Source: CAD feature listing. Evaluate the final solid. Frame: model axes, mm. A direction names the side the tool comes from. Round coordinates to 2 decimals unless told otherwise and drop trailing zeros. Loops run counter-clockwise (first coordinate to the right, second up) from the corner with the lowest first, then second, coordinate; pieces in that order, holes last. Notation, with made-up numbers: M 11.25,84.5 L 60.25,84.5 A23 ccw 60.25,99.5 Z; hole C 86.5,19 d6. An arc over 180 degrees is marked long. Answer as CSV lines item,"result". Start each with the question number.
```python
from build123d import *

# Parameters (mm, degrees)
SKETCH2_W           = 51.27
SKETCH2_H           = 26.65
BOSS_EXTRUDE2_DEPTH = 5
SKETCH3_W           = 45.27
SKETCH3_H           = 20.65
CUT_EXTRUDE1_DEPTH  = 6
SKETCH4_W           = 3.75
SKETCH4_H           = 3.75
BOSS_EXTRUDE3_DEPTH = 5
SKETCH5_R           = 1.12
CUT_EXTRUDE2_DEPTH  = 6
SKETCH6_W           = 15
SKETCH6_H           = 57.7
BOSS_EXTRUDE4_DEPTH = 5
SKETCH7_W           = 25.4
SKETCH7_H           = 9.5
BOSS_EXTRUDE5_DEPTH = 5
SKETCH11_R          = 1.75
CUT_EXTRUDE5_DEPTH  = 6
SKETCH12_W          = 25.4
SKETCH12_H          = 0.2
CUT_EXTRUDE6_DEPTH  = 6


with BuildPart() as part:
    # Sketch2 → Boss-Extrude2 (new body)
    with BuildSketch(Plane(origin=(0, 0, 0), x_dir=(1, 0, 0), z_dir=(0, 1, 0))):
        with Locations((22.635, 10.325)):
            Rectangle(SKETCH2_W, SKETCH2_H)
    extrude(amount=BOSS_EXTRUDE2_DEPTH)

    # Sketch3 → Cut-Extrude1 (cut, through all)
    with BuildSketch(Plane(origin=(0, 5, 0), x_dir=(1, 0, 0), z_dir=(0, 1, 0))):
        with Locations((22.635, 10.325)):
            Rectangle(SKETCH3_W, SKETCH3_H)
    extrude(amount=-CUT_EXTRUDE1_DEPTH, mode=Mode.SUBTRACT)

    # Sketch4 → Boss-Extrude3 (add)
    with BuildSketch(Plane(origin=(0, 5, 0), x_dir=(1, 0, 0), z_dir=(0, 1, 0))):
        with Locations((1.875, 18.775)):
            Rectangle(SKETCH4_W, SKETCH4_H)
        with Locations((1.875, 1.875)):
            Rectangle(SKETCH4_W, SKETCH4_H)
        with Locations((43.395, 1.875)):
            Rectangle(SKETCH4_W, SKETCH4_H)
        with Locations((43.395, 18.775)):
            Rectangle(SKETCH4_W, SKETCH4_H)
    extrude(amount=-BOSS_EXTRUDE3_DEPTH)

    # Sketch5 → Cut-Extrude2 (cut, through all)
    with BuildSketch(Plane(origin=(0, 5, 0), x_dir=(1, 0, 0), z_dir=(0, 1, 0))):
        with Locations((1.385, 18.975)):
            Circle(SKETCH5_R)
        with Locations((43.885, 18.975)):
            Circle(SKETCH5_R)
        with Locations((43.885, 1.675)):
            Circle(SKETCH5_R)
        with Locations((1.385, 1.675)):
            Circle(SKETCH5_R)
    extrude(amount=-CUT_EXTRUDE2_DEPTH, mode=Mode.SUBTRACT)

    # Sketch6 → Boss-Extrude4 (add)
    with BuildSketch(Plane(origin=(0, 5, 0), x_dir=(1, 0, 0), z_dir=(0, 1, 0))):
        with Locations((22.635, -31.85)):
            Rectangle(SKETCH6_W, SKETCH6_H)
    extrude(amount=-BOSS_EXTRUDE4_DEPTH)

    # Sketch7 → Boss-Extrude5 (add)
    with BuildSketch(Plane(origin=(0, 5, 0), x_dir=(1, 0, 0), z_dir=(0, 1, 0))):
        with Locations((22.635, -65.45)):
            Rectangle(SKETCH7_W, SKETCH7_H)
    extrude(amount=-BOSS_EXTRUDE5_DEPTH)

    # Sketch11 → Cut-Extrude5 (cut, through all)
    with BuildSketch(Plane.XZ):
        with Locations((30.335, 65.51777032)):
            Circle(SKETCH11_R)
        with Locations((14.935, 65.51777032)):
            Circle(SKETCH11_R)
    extrude(amount=-CUT_EXTRUDE5_DEPTH, mode=Mode.SUBTRACT)

    # Sketch12 → Cut-Extrude6 (cut, through all)
    with BuildSketch(Plane(origin=(0, 5, 0), x_dir=(1, 0, 0), z_dir=(0, 1, 0))):
        with Locations((22.635, -70.1)):
            Rectangle(SKETCH12_W, SKETCH12_H)
    extrude(amount=-CUT_EXTRUDE6_DEPTH, mode=Mode.SUBTRACT)


solid = part.part
```
1) Section C-C, the plane x = 40.5. Return loops of the section in (y, z), and give its area (3 significant figures).
2) Ray query, line 1 along Z through (x, y) = (10, 2.4); line 2 along Z through (x, y) = (4.5, 4.2); line 3 along Z through (x, y) = (3, 0.95). Return the intervals inside material, ascending.
3) Section A-A, the plane x = 26.5. Return loops of the section in (y, z), and give its area (3 significant figures).
4) Mould query, pull axis X, two halves, no side actions, for faces 5 (the flat face through (3.75, 3, -2)), 6 (the cylindrical face through (1.239, 2.535, -20.085)), 7 (the flat face through (22, 0, 23)), 8 (the flat face through (30.135, 3, 32)). Classes: pulls with the +X half, pulls with the -X half, needs draft (parallel to the pull), parting line crosses it, or undercut.
5) Contact query for flat-ended pins moving along their axis: pin 1 Ø3 at (y, z) = (2, 15) entering from -X (3 decimals); pin 2 Ø1.5 at (y, z) = (2, 67.5) entering from +X (3 decimals); pin 3 Ø12 at (x, z) = (23.5, -10) entering from -Y; pin 4 Ø1.5 at (y, z) = (1.5, 45.5) entering from +X (3 decimals). Output: stop coordinate, or through.
6) Section B-B, the plane y = 2.4. Give the number of separate pieces and of enclosed holes in the cut face, and give its area (3 significant figures).
7) Access query for faces 1 (the flat face through (35.335, 3, 65)), 2 (the flat face through (33, 3, 60.7)), 3 (the flat face through (9.935, 3, 65)), 4 (the flat face through (2, 3, -16.9)). Directions: +Z, -Z, +X, -X, +Y, -Y. A direction counts if a zero-diameter tool reaches every point of the face in a straight line with its end or side. Return the directions, or none.
8) Section D-D, the plane z = 9.5. Return loops of the section in (x, y) (3 decimals).
Findings below:
1,outline,"M 0,-23.65 L 5,-23.65 L 5,-20.65 L 0,-20.65 Z; M 0,0 L 5,0 L 5,3 L 0,3 Z"
1,area,"30.0 mm²"
2,line 1,"-23.65 to -20.65, 0 to 3, 60.7 to 70"
2,line 2,"-23.65 to -20.65, 0 to 3"
2,line 3,"-23.65 to -16.9, -3.75 to 3"
3,outline,"M 0,-23.65 L 5,-23.65 L 5,-20.65 L 0,-20.65 Z; M 0,0 L 5,0 L 5,70 L 0,70 Z"
3,area,"365 mm²"
4,face 5,"undercut"
4,face 6,"undercut"
4,face 7,"needs draft"
4,face 8,"pulls with the +X half"
5,pin 1,"x = 15.135"
5,pin 2,"x = 35.335"
5,pin 3,"through"
5,pin 4,"x = 30.135"
6,separate pieces,"1"
6,enclosed holes,"7"
6,area,"1,550 mm²"
7,face 1,"+Z, +X, +Y, -Y"
7,face 2,"+X, +Y, -Y"
7,face 3,"+Z, -X, +Y, -Y"
7,face 4,"+Y, -Y"
8,outline,"M 15.135,0 L 30.135,0 L 30.135,5 L 15.135,5 Z"
